For this review, take the finished solid that the model builds, in its own axes (mm). A direction names the side the tool comes from. Round coordinates to 2 decimals unless told otherwise and drop trailing zeros. Order: outer loops, then holes, each group sorted by start corner. A loop starts at its lowest first (then second) coordinate and runs counter-clockwise, first axis right, second up.
```python
from build123d import *

# Parameters (mm, degrees)
BOSS_EXTRUDE1_DEPTH = 10


with BuildPart() as part:
    # Sketch1 → Boss-Extrude1 (new body)
    with BuildSketch(Plane.XY):
        with BuildLine():
            Line((0, 4.980997276), (38.18012487, 4.980997276))
            Line((38.18012487, 4.980997276), (38.18012487, -24.126325443))
            Line((38.18012487, -24.126325443), (0, -24.126325443))
            Line((0, -24.126325443), (-13.14596048, -24.126325443))
            Line((-13.14596048, -24.126325443), (-13.14596048, -20))
            Line((-13.14596048, -20), (0, -20))
            ThreePointArc((0, -20), (10, -10), (0, 0))
            Line((0, 0), (-13.14596048, 0))
            Line((-13.14596048, 0), (-13.14596048, 4.980997276))
            Line((-13.14596048, 4.980997276), (0, 4.980997276))
        make_face()
    extrude(amount=BOSS_EXTRUDE1_DEPTH)


solid = part.part
```
Q1. Take a section at D-D, the plane y = -10. State the section outline as (x, z) points, plus the area to 3 significant figures.
Q2. Take a section at B-B, the plane z = 4.5. State the section outline as (x, y) points, plus the area to 3 significant figures.
Q3. Clearance check with a flat-ended pin moving along its axis: pin 1 (12 mm diameter, centred on x = -7, y = -12, fed in from -Z). State where the tip first meets the part, or that it passes through.
Q4. Tool access review of faces 1 (the face through (-7, -20, 5)), 2 (the face through (-13.146, -22, 5)): name each direction out of +Z, -Z, +X, -X, +Y, -Y from which nothing blocks a thin tool from reaching the whole face with its end or side.
Q5. Take a section at C-C, the plane y = -4. State the section outline as (x, z) points.
Q6. Wall thickness on line 1 (Y direction, x = -3, z = 5); line 2 (Y direction, x = 2, z = 9.5); line 3 (X direction, y = -17.25, z = 2.75): over which ranges is each line inside the solid? List them lowest first.
Q7. Mouldability with a two-part tool opening along Y and no side actions: class faces 3 (the face through (13, -24.126, 5)), 4 (the face through (10, -10, 5)), 5 (the face through (12, 4.981, 5)) as +Y half, -Y half, draft (parallel to the pull), parting line (faces both ways), or undercut.
Q8. Take a section at A-A, the plane x = -3.5. State the section outline as (y, z) points, plus the area to 3 significant figures.
Working result:
1. outline: (10, 0) - (38.18, 0) - (38.18, 10) - (10, 10) - close
1. area: 282 mm2
2. outline: (-13.15, -24.13) - (38.18, -24.13) - (38.18, 4.98) - (-13.15, 4.98) - (-13.15, 0) - (0, 0) arc R10 cw to (0, -20) - (-13.15, -20) - close
2. area: 1,070 mm2
3. pin 1: passes through
4. face 1: +Z, -Z, -X
4. face 2: +Z, -Z, -X, +Y, -Y
5. outline: (8, 0) - (38.18, 0) - (38.18, 10) - (8, 10) - close
6. line 1: y = -24.13 to -20, 0 to 4.98
6. line 2: y = -24.13 to -19.8, -0.2 to 4.98
6. line 3: x = 6.89 to 38.18
7. face 3: -Y half
7. face 4: undercut
7. face 5: +Y half
8. outline: (-24.13, 0) - (-20, 0) - (-20, 10) - (-24.13, 10) - close; (0, 0) - (4.98, 0) - (4.98, 10) - (0, 10) - close
8. area: 91.1 mm2
